from build123d import *

# Parameters (mm, degrees)
SKETCH1_W           = 85
SKETCH1_H           = 35
SKETCH1_R           = 1.5
BOSS_EXTRUDE2_DEPTH = 1.53
SKETCH2_W           = 71
SKETCH2_H           = 7.47
SKETCH2_W_2         = 5.75
SKETCH2_H_2         = 14.97
SKETCH2_W_3         = 11.74
SKETCH2_W_4         = 47.48
SKETCH2_H_3         = 12.47
BOSS_EXTRUDE3_DEPTH = 7


with BuildPart() as part:
    # Sketch1 → Boss-Extrude2 (new body)
    with BuildSketch(Plane(origin=(0, 0, 0), x_dir=(1, 0, 0), z_dir=(0, 1, 0))):
        Rectangle(SKETCH1_W, SKETCH1_H)
        with Locations(Location((-39.7, 14.5, 0), (0, 0, 270))):
            Circle(SKETCH1_R, mode=Mode.SUBTRACT)
        with Locations(Location((-39.7, -15, 0), (0, 0, 270))):
            Circle(SKETCH1_R, mode=Mode.SUBTRACT)
        with Locations(Location((40, 14.1, 0), (0, 0, 270))):
            Circle(SKETCH1_R, mode=Mode.SUBTRACT)
        with Locations(Location((40, -14.8, 0), (0, 0, 270))):
            Circle(SKETCH1_R, mode=Mode.SUBTRACT)
    extrude(amount=BOSS_EXTRUDE2_DEPTH)

    # Sketch2 → Boss-Extrude3 (add)
    with BuildSketch(Plane(origin=(0, 1.53, 0), x_dir=(1, 0, 0), z_dir=(0, 1, 0))):
        with Locations((-0.5, -13.765)):
            Rectangle(SKETCH2_W, SKETCH2_H)
        with Locations((32.125, 0.115)):
            Rectangle(SKETCH2_W_2, SKETCH2_H_2)
        with Locations((-30.13, 13.685)):
            Rectangle(SKETCH2_W_3, SKETCH2_H)
        with Locations((11.26, 13.685)):
            Rectangle(SKETCH2_W_4, SKETCH2_H)
        with Locations((-33.125, -1.135)):
            Rectangle(SKETCH2_W_2, SKETCH2_H_3)
    extrude(amount=BOSS_EXTRUDE3_DEPTH)


solid = part.part
Check sheet for the modelled part. Datum: model origin and axes. Units: mm. A direction names the side the tool comes from. Round coordinates to 2 decimals unless told otherwise and drop trailing zeros. Loops run counter-clockwise (first coordinate to the right, second up) from the corner with the lowest first, then second, coordinate; pieces in that order, holes last. Notation, with made-up numbers: (-1.75, -2.75) - (26.25, -2.75) arc R17 ccw to (26.25, 26.25) - close; hole circle Ø8 at (-1, 52.5). An arc over 180 degrees is marked (long way). Answer as CSV lines item,"result". Start each with the question number.
Item 1: Section check C-C (z = 15). Record the boundary of the cut face in (x, y), and give its area (3 significant figures).
Item 2: Section check B-B (x = 40). Record the boundary of the cut face in (y, z).
Item 3: Set-up check for faces 1 (the flat face through (29.25, 5, 0)), 2 (the flat face through (32, 5, -7.6)), 3 (the flat face through (-36, 5, 1)), 4 (the flat face through (-33, 5, -5.1)): record each of +Z, -Z, +X, -X, +Y, -Y from which the full face is reachable in a straight line by a thin tool's end or side.
Item 4: Depth check by flat-ended pin: P1, Ø5, axis at x = 40, z = -14.1, coming from the +Y side; P2, Ø2, axis at y = 4, z = -13.5, coming from the -X side; P3, Ø2, axis at y = 5.5, z = 14.5, coming from the +X side; P4, Ø2.5, axis at x = -39.7, z = 15, coming from the +Y side. Enter the tip coordinate at first touch or a pass-through.
Item 5: Section check A-A (y = 5.5). Record the boundary of the cut face in (x, z), and give its area (3 significant figures).
Item 6: Release check for a two-part mould opening along Z. For faces 5 (the flat face through (-30, 5, -17.42)), 6 (the cylindrical face through (-38.69, 0.75, -15.61)), 7 (the flat face through (-12.48, 5, -14)) record: +Z half, -Z half, draft (parallel to the pull), parting line (faces both ways), or undercut.
Item 7: Section check D-D (z = 11). Record the boundary of the cut face in (x, y).
Item 8: Scan lines: line 1 (X direction, y = 1.15, z = 15); line 2 (Z direction, x = 33.5, y = 6.75); line 3 (Z direction, x = -32, y = 4.75). Record each from-to range of solid material in increasing order. Write a range as [from, to].
Report:
1,outline,"(-42.5, 0) - (-41.2, 0) - (-41.2, 1.53) - (-42.5, 1.53) - close; (-38.2, 0) - (38.51, 0) - (38.51, 1.53) - (35, 1.53) - (35, 8.53) - (-36, 8.53) - (-36, 1.53) - (-38.2, 1.53) - close; (41.49, 0) - (42.5, 0) - (42.5, 1.53) - (41.49, 1.53) - close"
1,area,"618 mm2"
2,outline,"(0, -17.5) - (1.53, -17.5) - (1.53, -15.6) - (0, -15.6) - close; (0, -12.6) - (1.53, -12.6) - (1.53, 13.3) - (0, 13.3) - close; (0, 16.3) - (1.53, 16.3) - (1.53, 17.5) - (0, 17.5) - close"
3,face 1,"+Y"
3,face 2,"+X, -X, +Y"
3,face 3,"+Z, -Z, -X, +Y"
3,face 4,"-X, +Y"
4,P1,"stops at y = 1.53"
4,P2,"stops at x = -36"
4,P3,"stops at x = 35"
4,P4,"passes through"
5,outline,"(-36, -17.42) - (-24.26, -17.42) - (-24.26, -9.95) - (-36, -9.95) - close; (-36, -5.1) - (-30.25, -5.1) - (-30.25, 7.37) - (-36, 7.37) - close; (-36, 10.03) - (35, 10.03) - (35, 17.5) - (-36, 17.5) - close; (-12.48, -17.42) - (35, -17.42) - (35, -9.95) - (-12.48, -9.95) - close; (29.25, -7.6) - (35, -7.6) - (35, 7.37) - (29.25, 7.37) - close"
5,area,"1,130 mm2"
6,face 5,"-Z half"
6,face 6,"undercut"
6,face 7,"draft"
7,outline,"(-42.5, 0) - (42.5, 0) - (42.5, 1.53) - (35, 1.53) - (35, 8.53) - (-36, 8.53) - (-36, 1.53) - (-42.5, 1.53) - close"
8,line 1,"x = [-42.5, -41.2], [-38.2, 38.51], [41.49, 42.5]"
8,line 2,"z = [-17.42, -9.95], [-7.6, 7.37], [10.03, 17.5]"
8,line 3,"z = [-17.42, -9.95], [-5.1, 7.37], [10.03, 17.5]"
